Autodesk Inventor part; units mm, degrees
ref_plane "tnut_XY" through (0, 0, -1.2065) normal (0, 0, 1) x (1, 0, 0)
ref_plane "tnut_YZ" through (0, 0, -1.2065) normal (1, 0, 0) x (0, 1, 0)
ref_plane "tnut_ZX" through (0, 0, -1.2065) normal (0, 1, 0) x (0, 0, 1)
sketch "Sketch_1" plane through (0, 0, 0) normal (0, 0, 1) x (1, 0, 0)
  arc A0 (-5.6261, 5.6261) -> (-5.6261, -5.6261) centre (-5.6261, 0) ccw
  line L0 (-5.6261, -5.6261) -> (30.7467, -5.6261)
  arc A1 (30.7467, -5.6261) -> (30.7467, 5.6261) centre (30.7467, 0) ccw
  line L1 (30.7467, 5.6261) -> (-5.6261, 5.6261)
extrude "Extrusion1" add sketch "Sketch_1" along normal mid plane 2.413
sketch "Sketch_2" plane through (0, 0, 0) normal (0, 1, 0) x (-1, 0, 0)
  line L0 (0, 2.4765) -> (0, -1.2065)
  line L1 (0, -1.2065) -> (-3.7719, -1.2065)
  line L2 (-3.7719, -1.2065) -> (-3.7719, 2.4765)
  line L3 (-3.7719, 2.4765) -> (0, 2.4765)
  line L4 (0, 2.4765) -> (0, -1.2065)
revolve "Revolution1" add sketch "Sketch_2" angle 360 about axis through (0, 0, 2.4765) along (0, 0, 1)
sketch "Sketch_3" plane through (0, 0, 0) normal (0, 1, 0) x (-1, 0, 0)
  line L0 (-25.4, 2.4765) -> (-25.4, -1.2065)
  line L1 (-25.4, -1.2065) -> (-29.1719, -1.2065)
  line L2 (-29.1719, -1.2065) -> (-29.1719, 2.4765)
  line L3 (-29.1719, 2.4765) -> (-25.4, 2.4765)
  line L4 (-25.4, 2.4765) -> (-25.4, -1.2065)
revolve "Revolution2" add sketch "Sketch_3" angle 360 about axis through (25.4, 0, 2.4765) along (0, 0, 1)
sketch "Sketch_4" plane through (0, 0, 0) normal (0, 1, 0) x (-1, 0, 0)
  line L0 (0, 2.4765) -> (0, -1.2065)
  line L1 (0, -1.2065) -> (-3.175, -1.2065)
  line L2 (-3.175, -1.2065) -> (-2.4879, -0.5194)
  line L3 (-2.4879, -0.5194) -> (-2.4879, 1.7894)
  line L4 (-2.4879, 1.7894) -> (-3.175, 2.4765)
  line L5 (-3.175, 2.4765) -> (0, 2.4765)
  line L6 (0, 2.4765) -> (0, -1.2065)
revolve "Revolution3" cut sketch "Sketch_4" angle 360 about axis through (0, 0, 2.4765) along (0, 0, 1)
thread "Thread1"
sketch "Sketch_5" plane through (0, 0, 0) normal (0, 1, 0) x (-1, 0, 0)
  line L0 (-25.4, 2.4765) -> (-25.4, -1.2065)
  line L1 (-25.4, -1.2065) -> (-28.575, -1.2065)
  line L2 (-28.575, -1.2065) -> (-27.8879, -0.5194)
  line L3 (-27.8879, -0.5194) -> (-27.8879, 1.7894)
  line L4 (-27.8879, 1.7894) -> (-28.575, 2.4765)
  line L5 (-28.575, 2.4765) -> (-25.4, 2.4765)
  line L6 (-25.4, 2.4765) -> (-25.4, -1.2065)
revolve "Revolution4" cut sketch "Sketch_5" angle 360 about axis through (25.4, 0, 2.4765) along (0, 0, 1)
thread "Thread2"
ref_plane "tnut_XY" through (0, 0, -1.2065) normal (0, 0, 1) x (1, 0, 0)
ref_plane "tnut_YZ" through (0, 0, -1.2065) normal (1, 0, 0) x (0, 1, 0)
ref_plane "tnut_ZX" through (0, 0, -1.2065) normal (0, 1, 0) x (0, 0, 1)
ref_plane "tnut1_XY" through (25.4, 0, -1.2065) normal (0, 0, 1) x (1, 0, 0)
ref_plane "tnut1_YZ" through (25.4, 0, -1.2065) normal (1, 0, 0) x (0, 1, 0)
ref_plane "tnut1_ZX" through (25.4, 0, -1.2065) normal (0, 1, 0) x (0, 0, 1)
properties part number "3280"
Geometry check sheet. Reference: the model listing, model coordinates, mm. A direction names the side the tool comes from. Give positions to 0.01 mm unless a question says otherwise; leave off trailing zeros. Order: outer loops, then holes, each group sorted by start corner. A loop starts at its lowest first (then second) coordinate and runs counter-clockwise, first axis right, second up. Notation, with made-up numbers: (23.25, 80) - (80.25, 80) arc R8 cw to (80.25, 91) - close; hole circle Ø2 at (60.5, 35.25). An arc over 180 degrees is marked (long way). Answer as a JSON object with one key per item and string values.
(1) Tool access check on faces 1 (the flat face through (12, 0, 1.206)), 2 (the flat face through (13, 5.626, 0)). Record the directions out of +Z, -Z, +X, -X, +Y, -Y that give a thin tool (end or side, any length) a straight path to the whole face; none if there is none.
Report:
{"face 1": "+Z", "face 2": "+Z, -Z, +X, -X, +Y"}
(2) Cross-section at A-A (y = 0). Record the cut outline in (x, z) (1 decimal), then the cut area to 3 significant figures.
Report:
{"outline": "(-11.3, -1.2) - (-3.2, -1.2) - (-2.5, -0.5) - (-2.5, 1.8) - (-3.2, 2.5) - (-3.8, 2.5) - (-3.8, 1.2) - (-11.3, 1.2) - close; (2.5, -0.5) - (3.2, -1.2) - (22.2, -1.2) - (22.9, -0.5) - (22.9, 1.8) - (22.2, 2.5) - (21.6, 2.5) - (21.6, 1.2) - (3.8, 1.2) - (3.8, 2.5) - (3.2, 2.5) - (2.5, 1.8) - close; (27.9, -0.5) - (28.6, -1.2) - (36.4, -1.2) - (36.4, 1.2) - (29.2, 1.2) - (29.2, 2.5) - (28.6, 2.5) - (27.9, 1.8) - close", "area": "95.5 mm^2"}
(3) Cross-section at B-B (x = 25.4). Record the cut outline in (y, z) (1 decimal).
Report:
{"outline": "(-5.6, -1.2) - (-3.2, -1.2) - (-2.5, -0.5) - (-2.5, 1.8) - (-3.2, 2.5) - (-3.8, 2.5) - (-3.8, 1.2) - (-5.6, 1.2) - close; (2.5, -0.5) - (3.2, -1.2) - (5.6, -1.2) - (5.6, 1.2) - (3.8, 1.2) - (3.8, 2.5) - (3.2, 2.5) - (2.5, 1.8) - close"}
(4) Material ranges on line 1 (Y direction, x = 25.4, z = 1.3); line 2 (Y direction, x = 0, z = 0.9); line 3 (X direction, y = -1.5, z = -0.9), recorded low to high.
Report:
{"line 1": "-3.77 to -2.49, 2.49 to 3.77", "line 2": "-5.63 to -2.49, 2.49 to 5.63", "line 3": "-11.05 to -2.45, 2.45 to 22.95, 27.85 to 36.17"}
(5) Depth check by flat-ended pin: pin 1 Ø1.5 at (y, z) = (-2.5, 2) entering from +X; pin 2 Ø1 at (y, z) = (2, 1.5) entering from -X; pin 3 Ø5.5 at (x, y) = (25.4, 0) entering from +Z. Enter the tip coordinate at first touch or a pass-through.
Report:
{"pin 1": "x = 28.74", "pin 2": "x = -11.02", "pin 3": "z = 2.05"}
(6) Cross-section at D-D (y = 4.5). Record the cut outline in (x, z).
Report:
{"outline": "(-9, -1.21) - (34.12, -1.21) - (34.12, 1.21) - (-9, 1.21) - close"}
(7) Cross-section at C-C (x = 8). Record the cut outline in (y, z), then the cut area to 3 significant figures.
Report:
{"outline": "(-5.63, -1.21) - (5.63, -1.21) - (5.63, 1.21) - (-5.63, 1.21) - close", "area": "27.2 mm^2"}
(8) Draft check along X on faces 3 (the cylindrical face through (22.915, 0.109, 0.651)), 4 (the flat face through (12, -5.626, 0)), 5 (the cylindrical face through (-11.25, -0.12, -0.02)). Enter one of: released by +X, released by -X, zero draft, split by the parting line, or undercut.
Report:
{"face 3": "undercut", "face 4": "zero draft", "face 5": "released by -X"}
